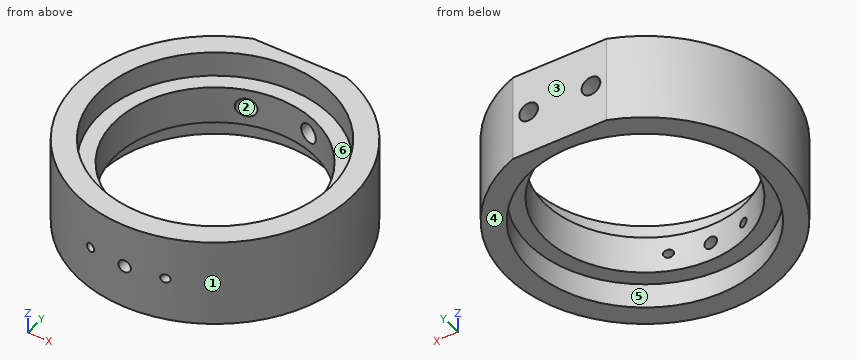
from build123d import *

# Parameters (mm, degrees)
SKETCH_1_R               = 22
SKETCH_1_R_2             = 18.5
EXTRUDE_1_DEPTH          = 10
EXTRUDE_START            = -6
SKETCH_2_R               = 18.5
SKETCH_2_R_2             = 16
EXTRUDE_2_DEPTH          = 6
CUT_EXTRUDE_3_DEPTH      = 33.680269277
CUT_EXTRUDE_4_REACH      = 51.049
CUT_EXTRUDE_4_END_RADIUS = 16
SKETCH_8_R               = 1.5
SKETCH_10_R              = 1
SKETCH_10_R_2            = 0.7
CUT_EXTRUDE_5_DEPTH      = 33.680269307
SKETCH_11_R              = 18.5
EXTRUDE_3_DEPTH          = 4


with BuildPart() as part:
    # 草图1 → 凸台-拉伸1 (new body)
    with BuildSketch(Plane.XY):
        Circle(SKETCH_1_R)
        Circle(SKETCH_1_R_2, mode=Mode.SUBTRACT)
    extrude(amount=EXTRUDE_1_DEPTH)

    # 草图2 → 凸台-拉伸2 (add)
    with BuildSketch(Plane.XY.offset(10).offset(EXTRUDE_START)):
        Circle(SKETCH_2_R)
        Circle(SKETCH_2_R_2, mode=Mode.SUBTRACT)
    extrude(amount=EXTRUDE_2_DEPTH)

    # 草图7 → 切除-拉伸3 (cut, through all)
    with BuildSketch(Plane.XY.offset(10)):
        with BuildLine():
            Line((-7.5, 20.68211788), (7.5, 20.68211788))
            ThreePointArc((7.5, 20.68211788), (0, 22), (-7.5, 20.68211788))
        make_face()
    extrude(amount=-CUT_EXTRUDE_3_DEPTH, mode=Mode.SUBTRACT)

    # 切除-拉伸4: up to this cylinder (the profile starts outside it)
    cut_extrude_4_end = Plane(origin=(0, 0, 7), z_dir=(0, 0, 1)) * Cylinder(CUT_EXTRUDE_4_END_RADIUS, 135.098, mode=Mode.PRIVATE)
    # 草图8 → 切除-拉伸4 (cut, up to the surface)
    with BuildSketch(Plane(origin=(0, 20.68211788, 0), x_dir=(1, 0, 0), z_dir=(0, 1, 0)), mode=Mode.PRIVATE) as cut_extrude_4_sk1:
        with Locations(Location((-5, -7, 0), (0, 0, 270))):
            Circle(SKETCH_8_R)
    cut_extrude_4_tool1 = extrude(cut_extrude_4_sk1.sketch, amount=-CUT_EXTRUDE_4_REACH, mode=Mode.PRIVATE) - cut_extrude_4_end
    add(cut_extrude_4_tool1.solids().sort_by_distance((-5, 20.682118, 7))[0], mode=Mode.SUBTRACT)
    # 草图8 → 切除-拉伸4 (cut, up to the surface)
    with BuildSketch(Plane(origin=(0, 20.68211788, 0), x_dir=(1, 0, 0), z_dir=(0, 1, 0)), mode=Mode.PRIVATE) as cut_extrude_4_sk2:
        with Locations(Location((5, -7, 0), (0, 0, 270))):
            Circle(SKETCH_8_R)
    cut_extrude_4_tool2 = extrude(cut_extrude_4_sk2.sketch, amount=-CUT_EXTRUDE_4_REACH, mode=Mode.PRIVATE) - cut_extrude_4_end
    add(cut_extrude_4_tool2.solids().sort_by_distance((5, 20.682118, 7))[0], mode=Mode.SUBTRACT)

    # 草图10 → 切除-拉伸5 (cut, through all)
    with BuildSketch(Plane(origin=(0, 0, 0), x_dir=(1, 0, 0), z_dir=(0, 1, 0))):
        with Locations(Location((0, -7, 0), (0, 0, 270))):
            Circle(SKETCH_10_R)
        with Locations(Location((-6, -7, 0), (0, 0, 270))):
            Circle(SKETCH_10_R_2)
        with Locations(Location((6, -7, 0), (0, 0, 270))):
            Circle(SKETCH_10_R_2)
    extrude(amount=-CUT_EXTRUDE_5_DEPTH, mode=Mode.SUBTRACT)

    # 草图11 → 凸台-拉伸3 (add)
    with BuildSketch(Plane.XY.offset(10)):
        with BuildLine():
            Line((-7.5, 20.68211788), (7.5, 20.68211788))
            ThreePointArc((7.5, 20.68211788), (0, -22), (-7.5, 20.68211788))
        make_face()
        Circle(SKETCH_11_R, mode=Mode.SUBTRACT)
    extrude(amount=EXTRUDE_3_DEPTH)


solid = part.part
Model file for the job. Use its own axes, mm. Face numbers are marked on the shaded views. A direction names the side the tool comes from. Give positions to 0.01 mm unless a question says otherwise; leave off trailing zeros. Order: outer loops, then holes, each group sorted by start corner. A loop starts at its lowest first (then second) coordinate and runs counter-clockwise, first axis right, second up. Notation, with made-up numbers: M 40.25,45 L 83.25,45 A16 ccw 83.25,70 Z; hole C -14.75,71 d4. An arc over 180 degrees is marked long. Write item = value, one per line.
Q1. Cut at B-B, the plane y = 3. List the corners of the cut face in (x, z).
Derived:
outline = M -21.79,0 L -18.26,0 L -18.26,4 L -15.72,4 L -15.72,10 L -18.26,10 L -18.26,14 L -21.79,14 Z; M 15.72,4 L 18.26,4 L 18.26,0 L 21.79,0 L 21.79,14 L 18.26,14 L 18.26,10 L 15.72,10 Z
Q2. Tool access for the marked faces 4, 5 and 6: list every direction of +Z, -Z, +X, -X, +Y, -Y with a clear straight run to the whole face (end or side of a thin tool).
Derived:
face_4 = -Z, +X, -X, +Y, -Y
face_5 = -Z
face_6 = +Z
Q3. Two-plate mould, pull along X, no slides. Class the marked faces 1, 2 and 3: pulls with the +X half, pulls with the -X half, needs draft (parallel to the pull), parting line crosses it, or undercut.
Derived:
face_1 = parting line crosses it
face_2 = undercut
face_3 = needs draft
Q4. Flat gauge pins, fed straight in: pin 1 (2 mm diameter, centred on x = -6, z = 7, fed in from -Y); pin 2 (1.5 mm diameter, centred on y = -10.5, z = 5, fed in from +X); pin 3 (2 mm diameter, centred on x = 15.5, z = 4, fed in from +Y). Where does each tip first touch, or does it go through?
Derived:
pin_1 = -21.42
pin_2 = 19.72
pin_3 = 16.55
Q5. Drill centre lines: line 1 (Z direction, x = 5, y = 17); line 2 (Y direction, x = 0, z = 12.95); line 3 (Z direction, x = -5, y = 18.25). Where is each one in solid material? Low to high. Write a range as [from, to].
Derived:
line_1 = [4, 5.5], [8.5, 10]
line_2 = [-22, -18.5], [18.5, 20.68]
line_3 = [0, 5.5], [8.5, 14]
Q6. Cut at D-D, the plane z = 7. List the corners of the cut face in (x, y).
Derived:
outline = M -7.5,20.68 A22 ccw -6.7,-20.95 L -6.7,-14.53 A16 cw -6.5,14.62 L -6.5,20.68 Z; M -5.3,-21.35 A22 ccw -1,-21.98 L -1,-15.97 A16 cw -5.3,-15.1 Z; M -3.5,15.61 A16 cw 3.5,15.61 L 3.5,20.68 L -3.5,20.68 Z; M 1,-21.98 A22 ccw 5.3,-21.35 L 5.3,-15.1 A16 cw 1,-15.97 Z; M 6.5,14.62 A16 cw 6.7,-14.53 L 6.7,-20.95 A22 ccw 7.5,20.68 L 6.5,20.68 Z
Q7. Cut at A-A, the plane x = 0. List the corners of the cut face in (y, z), then the cut area to 3 significant figures.
Derived:
outline = M -22,0 L -18.5,0 L -18.5,4 L -16,4 L -16,6 L -22,6 Z; M -22,8 L -16,8 L -16,10 L -18.5,10 L -18.5,14 L -22,14 Z; M 16,4 L 18.5,4 L 18.5,0 L 20.68,0 L 20.68,14 L 18.5,14 L 18.5,10 L 16,10 Z
area = 97.5 mm2
Q8. Cut at C-C, the plane x = 11. List the corners of the cut face in (y, z).
Derived:
outline = M -19.05,0 L -14.87,0 L -14.87,4 L -11.62,4 L -11.62,10 L -14.87,10 L -14.87,14 L -19.05,14 Z; M 11.62,4 L 14.87,4 L 14.87,0 L 19.05,0 L 19.05,14 L 14.87,14 L 14.87,10 L 11.62,10 Z
